The drawing under review shows one solid part. Ordinate dimensions are in mm from its lowest x, y, z. Coordinates: 2 decimals unless noted, no trailing zeros. Order: outer loops, then holes, each group sorted by start corner. A loop starts at its lowest first (then second) coordinate and runs counter-clockwise, first axis right, second up. Notation, with made-up numbers: (-27.5, -11) - (-13.5, -11) arc R30 cw to (-13.5, 16) - close; hole circle Ø1 at (18.5, -3.5). An arc over 180 degrees is marked (long way). Write each question's results on one line, items separated by ' | '. Start each with the question number.
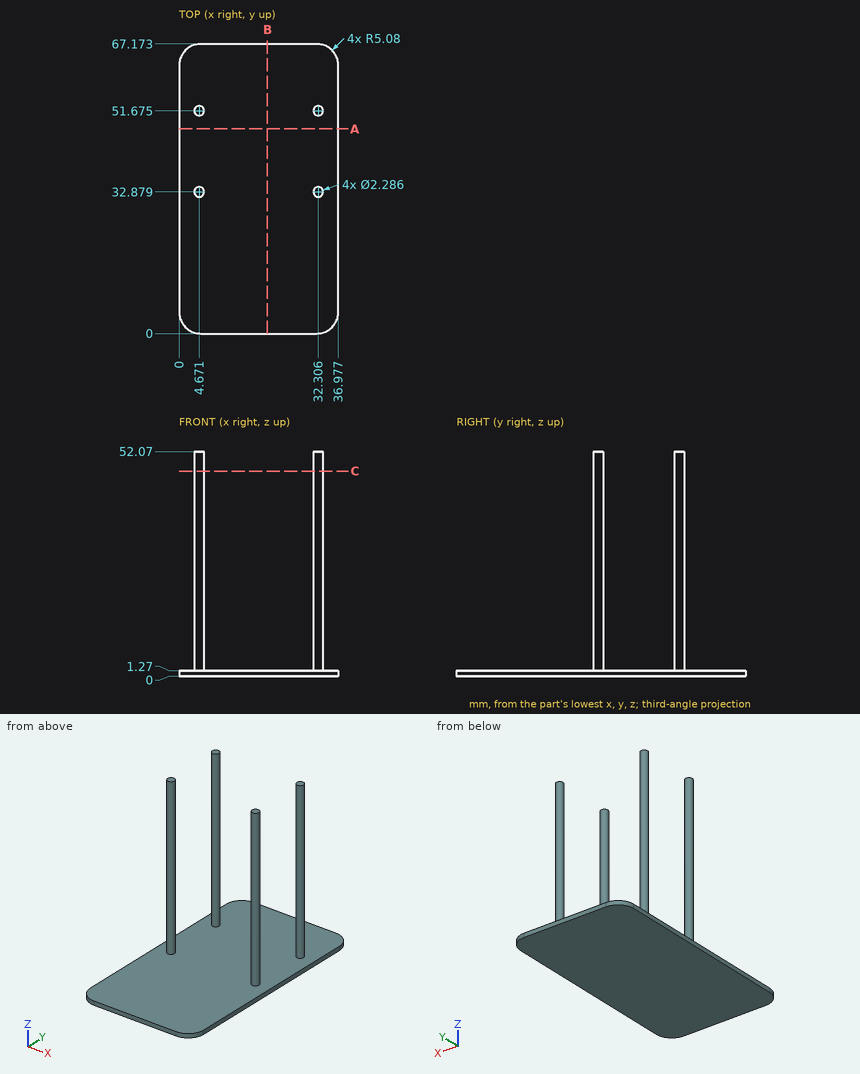
(1) Take a section at C-C (z = 47.5). State how many separate pieces and enclosed holes the cut face has, plus the area to 3 significant figures.
(2) Take a section at A-A (y = 47.5). State the section outline as (x, z) points.
(3) To check wall thickness, follow line 1 along Z through (x, y) = (28, 23); line 2 along X through (y, z) = (52, 22.5) (1 decimal). State the ranges of each line that lie inside material, in increasing order. Write a range as [from, to].
(4) Take a section at B-B (x = 20.5). State the section outline as (y, z) points.
(5) Clearance check with flat-ended pins moving along their axes: pin 1 (10 mm diameter, centred on x = 32.5, z = 10, fed in from -Y); pin 2 (12 mm diameter, centred on y = 26, z = 32.5, fed in from -X); pin 3 (10 mm diameter, centred on x = 15, y = 31, fed in from +Z). State where each tip first meets the part, or that it passes through.
Worked out:
1) separate pieces: 4 | enclosed holes: 0 | area: 16.4 mm^2
2) outline: (0, 0) - (36.98, 0) - (36.98, 1.27) - (0, 1.27) - close
3) line 1: [0, 1.27] | line 2: [3.6, 5.8], [31.2, 33.4]
4) outline: (0, 0) - (67.17, 0) - (67.17, 1.27) - (0, 1.27) - close
5) pin 1: y = 31.74 | pin 2: x = 3.94 | pin 3: z = 1.27
